Check sheet for the modelled part. Datum: model origin and axes. Units: mm. A direction names the side the tool comes from. Coordinates: 2 decimals unless noted, no trailing zeros. Loops run counter-clockwise (first coordinate to the right, second up) from the corner with the lowest first, then second, coordinate; pieces in that order, holes last. Notation, with made-up numbers: M 38.5,28.25 L 92.5,28.25 A19 ccw 92.5,51.25 Z; hole C 25,87 d5. An arc over 180 degrees is marked long. Answer in a Markdown table with one row per item. Add a question column.
```python
from build123d import *

# Parameters (mm, degrees)
SKETCH1_W                         = 57
SKETCH1_H                         = 57
MOTOR_RECTANGULAR_FRAME_DEPTH     = 112
MOTOR_SCREW_HOLE_LENGTHS_DEPTH    = 106.5
SKETCH3_R                         = 2.55
MOTOR_MOUNT_HOLES_DEPTH           = 114.87163826
SKETCH4_R                         = 6
REAR_BEARING_AND_SHAFT_DEPTH      = 4.5
SKETCH5_R                         = 6
SKETCH5_R_2                       = 4.5
REAR_BEARING_SHIELD_DEPTH         = 0.5
SKETCH6_R                         = 8
HOLLOWED_SECTION_REAR_DEPTH       = 3
SKETCH7_R                         = 19.05
FRONT_PLATFORM_EXTRUDE_DEPTH      = 1.6
FRONT_START                       = -3
SKETCH8_R                         = 6
FRONT_BEARING_DEPTH               = 3
FRONT_SHAFT_DEPTH                 = 21
FRONT_START_2                     = -0.5
SKETCH10_R                        = 6
SKETCH10_R_2                      = 5.25
FRONT_BEARING_SHEILD_DEPTH        = 0.5
MOTOR_SHAFT_CHAMFER_SIZE          = 0.5
MOTOR_FRONT_EDGE_FILLET_R         = 3
FRONT_COVER_SCREW_INDENTS_DEPTH   = 3
FRONT_COVER_SCREW_INDENT_FILLET_R = 1
SKETCH12_W                        = 7
SKETCH12_H                        = 5
SKETCH12_W_2                      = 5
SKETCH12_H_2                      = 4
WIRE_AREA_DEPTH                   = 3


with BuildPart() as part:
    # Sketch1 → Motor rectangular frame (new body)
    with BuildSketch(Plane(origin=(0, 0, 0), x_dir=(1, 0, 0), z_dir=(0, 1, 0))):
        Rectangle(SKETCH1_W, SKETCH1_H)
    extrude(amount=MOTOR_RECTANGULAR_FRAME_DEPTH)

    # Sketch2 → Motor screw hole lengths (cut)
    with BuildSketch(Plane.XZ):
        with BuildLine():
            Line((-26.5, 19.5), (-21.5, 19.5))
            ThreePointArc((-21.5, 19.5), (-20.085786438, 20.085786438), (-19.5, 21.5))
            Line((-19.5, 21.5), (-19.5, 26.5))
            ThreePointArc((-19.5, 26.5), (-18.914213562, 27.914213562), (-17.5, 28.5))
            Line((-17.5, 28.5), (-28.5, 28.5))
            Line((-28.5, 28.5), (-28.5, 17.5))
            ThreePointArc((-28.5, 17.5), (-27.914213562, 18.914213562), (-26.5, 19.5))
        make_face()
        with BuildLine():
            Line((19.5, 26.5), (19.5, 21.5))
            ThreePointArc((19.5, 21.5), (20.085786438, 20.085786438), (21.5, 19.5))
            Line((21.5, 19.5), (26.5, 19.5))
            ThreePointArc((26.5, 19.5), (27.914213562, 18.914213562), (28.5, 17.5))
            Line((28.5, 17.5), (28.5, 28.5))
            Line((28.5, 28.5), (17.5, 28.5))
            ThreePointArc((17.5, 28.5), (18.914213562, 27.914213562), (19.5, 26.5))
        make_face()
        with BuildLine():
            Line((26.5, -19.5), (21.5, -19.5))
            ThreePointArc((21.5, -19.5), (20.085786438, -20.085786438), (19.5, -21.5))
            Line((19.5, -21.5), (19.5, -26.5))
            ThreePointArc((19.5, -26.5), (18.914213562, -27.914213562), (17.5, -28.5))
            Line((17.5, -28.5), (28.5, -28.5))
            Line((28.5, -28.5), (28.5, -17.5))
            ThreePointArc((28.5, -17.5), (27.914213562, -18.914213562), (26.5, -19.5))
        make_face()
        with BuildLine():
            Line((-19.5, -26.5), (-19.5, -21.5))
            ThreePointArc((-19.5, -21.5), (-20.085786438, -20.085786438), (-21.5, -19.5))
            Line((-21.5, -19.5), (-26.5, -19.5))
            ThreePointArc((-26.5, -19.5), (-27.914213562, -18.914213562), (-28.5, -17.5))
            Line((-28.5, -17.5), (-28.5, -28.5))
            Line((-28.5, -28.5), (-17.5, -28.5))
            ThreePointArc((-17.5, -28.5), (-18.914213562, -27.914213562), (-19.5, -26.5))
        make_face()
    extrude(amount=-MOTOR_SCREW_HOLE_LENGTHS_DEPTH, mode=Mode.SUBTRACT)

    # Sketch3 → Motor mount holes (cut, through all)
    with BuildSketch(Plane.XZ.offset(-106.5)):
        with Locations(Location((-23.57, 23.57, 0), (0, 0, 270))):
            Circle(SKETCH3_R)
        with Locations(Location((23.57, 23.57, 0), (0, 0, 270))):
            Circle(SKETCH3_R)
        with Locations(Location((23.57, -23.57, 0), (0, 0, 90))):
            Circle(SKETCH3_R)
        with Locations(Location((-23.57, -23.57, 0), (0, 0, 90))):
            Circle(SKETCH3_R)
    extrude(amount=-MOTOR_MOUNT_HOLES_DEPTH, mode=Mode.SUBTRACT)

    # Sketch4 → Rear bearing and shaft (cut)
    with BuildSketch(Plane.XZ):
        with Locations(Location((0, 0, 0), (0, 0, 270))):
            Circle(SKETCH4_R)
    extrude(amount=-REAR_BEARING_AND_SHAFT_DEPTH, mode=Mode.SUBTRACT)

    # Sketch5 → Rear bearing shield (cut)
    with BuildSketch(Plane.XZ.offset(-4.5)):
        with Locations(Location((0, 0, 0), (0, 0, 270))):
            Circle(SKETCH5_R)
        with Locations(Location((0, 0, 0), (0, 0, 270))):
            Circle(SKETCH5_R_2, mode=Mode.SUBTRACT)
    extrude(amount=-REAR_BEARING_SHIELD_DEPTH, mode=Mode.SUBTRACT)

    # Sketch6 → Hollowed section (rear) (cut)
    with BuildSketch(Plane.XZ.offset(-4.5)):
        with Locations(Location((0, 0, 0), (0, 0, 270))):
            Circle(SKETCH6_R)
    extrude(amount=HOLLOWED_SECTION_REAR_DEPTH, mode=Mode.SUBTRACT)

    # Sketch7 → Front platform extrude (add)
    with BuildSketch(Plane(origin=(0, 112, 0), x_dir=(1, 0, 0), z_dir=(0, 1, 0))):
        with Locations(Location((0, 0, 0), (0, 0, 270))):
            Circle(SKETCH7_R)
    extrude(amount=FRONT_PLATFORM_EXTRUDE_DEPTH)

    # Sketch8 → Front bearing (cut)
    with BuildSketch(Plane(origin=(0, 113.6, 0), x_dir=(1, 0, 0), z_dir=(0, 1, 0)).offset(FRONT_START)):
        with Locations(Location((0, 0, 0), (0, 0, 90))):
            Circle(SKETCH8_R)
    extrude(amount=FRONT_BEARING_DEPTH, mode=Mode.SUBTRACT)

    # Sketch9 → Front shaft (add)
    with BuildSketch(Plane(origin=(0, 110.6, 0), x_dir=(1, 0, 0), z_dir=(0, 1, 0))):
        with BuildLine():
            Line((-1.936491673, 3.5), (1.936491673, 3.5))
            ThreePointArc((1.936491673, 3.5), (0, -4), (-1.936491673, 3.5))
        make_face()
    extrude(amount=FRONT_SHAFT_DEPTH)

    # Sketch10 → Front bearing sheild (cut)
    with BuildSketch(Plane(origin=(0, 110.6, 0), x_dir=(1, 0, 0), z_dir=(0, 1, 0)).offset(FRONT_START_2)):
        with Locations(Location((0, 0, 0), (0, 0, 90))):
            Circle(SKETCH10_R)
        with Locations(Location((0, 0, 0), (0, 0, 270))):
            Circle(SKETCH10_R_2, mode=Mode.SUBTRACT)
    extrude(amount=FRONT_BEARING_SHEILD_DEPTH, mode=Mode.SUBTRACT)

    # Motor shaft chamfer
    motor_shaft_chamfer_edges = [part.edges().sort_by_distance(p)[0] for p in [
        (0, 131.6, 4),
        (0, 131.6, -3.5),
    ]]
    chamfer(motor_shaft_chamfer_edges, length=MOTOR_SHAFT_CHAMFER_SIZE - 0.0001)  # a hair under: the kernel refuses the full size

    # Motor front edge fillet
    motor_front_edge_fillet_edges = [part.edges().sort_by_distance(p)[0] for p in [
        (28.5, 109.25, 28.5),
        (-28.5, 109.25, 28.5),
        (-28.5, 109.25, -28.5),
        (28.5, 109.25, -28.5),
    ]]
    fillet(motor_front_edge_fillet_edges, radius=MOTOR_FRONT_EDGE_FILLET_R)

    # Sketch11 → Front cover screw indents (cut)
    with BuildSketch(Plane(origin=(0, 112, 0), x_dir=(1, 0, 0), z_dir=(0, 1, 0))):
        with BuildLine():
            Line((26, 17.55), (28.5, 17.55))
            Line((28.5, 17.55), (28.5, 12.45))
            Line((28.5, 12.45), (26, 12.45))
            ThreePointArc((26, 12.45), (23.45, 15), (26, 17.55))
        make_face()
        with BuildLine():
            Line((26, -12.45), (28.5, -12.45))
            Line((28.5, -12.45), (28.5, -17.55))
            Line((28.5, -17.55), (26, -17.55))
            ThreePointArc((26, -17.55), (23.45, -15), (26, -12.45))
        make_face()
        with BuildLine():
            Line((-26, -12.45), (-28.5, -12.45))
            Line((-28.5, -12.45), (-28.5, -17.55))
            Line((-28.5, -17.55), (-26, -17.55))
            ThreePointArc((-26, -17.55), (-23.45, -15), (-26, -12.45))
        make_face()
        with BuildLine():
            Line((-26, 17.55), (-28.5, 17.55))
            Line((-28.5, 17.55), (-28.5, 12.45))
            Line((-28.5, 12.45), (-26, 12.45))
            ThreePointArc((-26, 12.45), (-23.45, 15), (-26, 17.55))
        make_face()
    extrude(amount=-FRONT_COVER_SCREW_INDENTS_DEPTH, mode=Mode.SUBTRACT)

    # Front cover screw indent fillet
    front_cover_screw_indent_fillet_edges = [part.edges().sort_by_distance(p)[0] for p in [
        (-28.5, 110.5, -12.45),
        (-28.5, 110.5, -17.55),
        (-23.45, 112, -15),
        (-27.25, 112, -17.55),
        (-27.25, 112, -12.45),
        (-28.5, 110.5, 17.55),
        (-28.5, 110.5, 12.45),
        (-23.45, 112, 15),
        (-27.25, 112, 12.45),
        (-27.25, 112, 17.55),
        (28.5, 110.5, 12.45),
        (28.5, 110.5, 17.55),
        (23.45, 112, 15),
        (27.25, 112, 17.55),
        (27.25, 112, 12.45),
        (28.5, 110.5, -17.55),
        (28.5, 110.5, -12.45),
        (23.45, 112, -15),
        (27.25, 112, -12.45),
        (27.25, 112, -17.55),
    ]]
    fillet(front_cover_screw_indent_fillet_edges, radius=FRONT_COVER_SCREW_INDENT_FILLET_R)

    # Sketch12 → Wire area (add)
    with BuildSketch(Plane(origin=(0, 0, -28.5), x_dir=(-1, 0, 0), z_dir=(0, 0, -1))):
        with Locations((0, 2.5)):
            Rectangle(SKETCH12_W, SKETCH12_H)
        with Locations((0, 2.5)):
            Rectangle(SKETCH12_W_2, SKETCH12_H_2, mode=Mode.SUBTRACT)
    extrude(amount=WIRE_AREA_DEPTH)


solid = part.part
```
Q1. Cross-section at C-C (x = 14.5). Record the cut outline in (y, z), plus the area to 3 significant figures.
Q2. Go/stop test with flat-tipped pins: pin 1 (4 mm diameter, centred on x = 25, y = 73, fed in from -Z); pin 2 (1.5 mm diameter, centred on y = 2.5, z = -30.5, fed in from +X); pin 3 (0.8 mm diameter, centred on x = -26.5, y = 110, fed in from +Z). Record where each tip stops, or that it passes through.
Q3. Cross-section at D-D (z = -15). Record the cut outline in (x, y).
Q4. Cross-section at B-B (y = 79.5). Record the cut outline in (x, z).
Q5. Access from +Z, -Z, +X, -X, +Y, -Y to the whole of each face (thin tool, end or side, straight path). Record for faces 5 (the face through (23.45, 110.01, 15.06)), 6 (the face through (24, 53, 19.5)), 7 (the face through (-0.4, 112, -19.4)), 8 (the face through (1.802, 4.746, -5.723)), 9 (the face through (24, 53, -19.5)).
Q6. Thickness scan on L1, parallel to X at y = 4.9, z = 0; L2, parallel to X at y = 3, z = 0; L3, parallel to Z at x = -23, y = 109. Record the ranges inside material, lowest first.
Q7. Mould release check, pull along X, two halves, no side actions. Record for faces 1 (the face through (3.5, 2, -30)), 2 (the face through (0, 55, 28.5)), 3 (the face through (22.593, 109.212, 21.214)), 4 (the face through (-1.802, 111.825, -5.723)): released by +X, released by -X, zero draft, split by the parting line, or undercut.
Q8. Cross-section at A-A (z = 23.57). Record the cut outline in (x, y), plus the area to 3 significant figures.
Answer key:
| question | item | result |
|---|---|---|
| 1 | outline | M 0,-28.5 L 112,-28.5 L 112,-12.36 L 113.6,-12.36 L 113.6,12.36 L 112,12.36 L 112,28.5 L 0,28.5 Z |
| 1 | area | 6,420 mm^2 |
| 2 | pin 1 | z = -19.5 |
| 2 | pin 2 | x = 3.5 |
| 2 | pin 3 | z = 28.44 |
| 3 | outline | M -28.5,0 L 28.5,0 L 28.5,109 L 23.45,109 L 23.45,111 A1 ccw 22.45,112 L 11.74,112 L 11.74,113.6 L -11.74,113.6 L -11.74,112 L -22.45,112 A1 ccw -23.45,111 L -23.45,109 L -28.5,109 Z |
| 4 | outline | M -28.5,-17.5 A2 ccw -26.5,-19.5 L -21.5,-19.5 A2 cw -19.5,-21.5 L -19.5,-26.5 A2 ccw -17.5,-28.5 L 17.5,-28.5 A2 ccw 19.5,-26.5 L 19.5,-21.5 A2 cw 21.5,-19.5 L 26.5,-19.5 A2 ccw 28.5,-17.5 L 28.5,17.5 A2 ccw 26.5,19.5 L 21.5,19.5 A2 cw 19.5,21.5 L 19.5,26.5 A2 ccw 17.5,28.5 L -17.5,28.5 A2 ccw -19.5,26.5 L -19.5,21.5 A2 cw -21.5,19.5 L -26.5,19.5 A2 ccw -28.5,17.5 Z |
| 5 | face 5 | +X, +Y |
| 5 | face 6 | +Z, +X, -Y |
| 5 | face 7 | +Y |
| 5 | face 8 | -Y |
| 5 | face 9 | -Z, +X, -Y |
| 6 | L1 | -28.5 to -6, -4.5 to 4.5, 6 to 28.5 |
| 6 | L2 | -28.5 to -8, 8 to 28.5 |
| 6 | L3 | -28.5 to -26.06, -21.08 to 21.08, 26.06 to 28.5 |
| 7 | face 1 | released by +X |
| 7 | face 2 | zero draft |
| 7 | face 3 | undercut |
| 7 | face 4 | undercut |
| 8 | outline | M -28.5,106.5 L -26.12,106.5 L -26.12,112 L -28.5,112 Z; M -21.02,106.5 L -19.5,106.5 L -19.5,0 L 19.5,0 L 19.5,106.5 L 21.02,106.5 L 21.02,112 L -21.02,112 Z; M 26.12,106.5 L 28.5,106.5 L 28.5,112 L 26.12,112 Z |
| 8 | area | 4,410 mm^2 |
